Autodesk Inventor part; units mm, degrees
ref_plane "YZ Plane" through (0, 0, 0) normal (1, 0, 0) x (0, 1, 0)
ref_plane "XZ Plane" through (0, 0, 0) normal (0, 1, 0) x (-1, 0, 0)
ref_plane "XY Plane" through (0, 0, 0) normal (0, 0, 1) x (1, 0, 0)
sketch "Sketch1" plane through (0, 0, 0) normal (0, 1, 0) x (-1, 0, 0)
  circle A0 centre (0, 0) radius 335
  dimension "d0" = 670
extrude "Extrusion1" add sketch "Sketch1" along normal blind 10
sketch "Sketch2" plane through (0, 10, 0) normal (0, 1, 0) x (1, 0, 0)
  circle A0 centre (-310, 0) radius 11
  circle A1 centre (0, 0) radius 310 construction
  dimension "d4" = 620
  dimension "d3" = 22
extrude "Cut1" cut sketch "Sketch2" against normal blind 10
pattern_circular "Circular Pattern1" count 20 over 360 about axis through (0, 0, 0) along (0, 1, 0) of "Cut1"
equation "\"d1\" = Thickness"
equation "\"d6\" = Thickness"
equation "\"BendReliefDepth\" = 0.5 * Thickness"
properties part number "PRS 1621 charging hatch D940"
Build history of the part. All positions in model axes, mm. Coordinates: 2 decimals unless noted, no trailing zeros. Write each loop counter-clockwise with the first axis right and the second up, starting at its lowest first coordinate (ties: lowest second). Pieces come first, ordered by that corner, then holes.
1. Band-saw the part on C-C, the plane y = 6.25. Give the number of separate pieces and of enclosed holes in the cut face, and give its area (3 significant figures).
Answer block:
separate pieces: 1
enclosed holes: 20
area: 345,000 mm2
2. Band-saw the part on B-B, the plane x = 0. Give the cut face in (y, z).
Answer block:
outline: (0, -335) - (10, -335) - (10, -321) - (0, -321) - close; (0, -299) - (10, -299) - (10, 299) - (0, 299) - close; (0, 321) - (10, 321) - (10, 335) - (0, 335) - close
3. Drill centre lines: probe 1 along Z at (x, y) = (256, 6.75); probe 2 along X at (y, z) = (4.75, 183.5); probe 3 along X at (y, z) = (8.25, 295.5). Where is each one in solid material? Low to high.
Answer block:
probe 1: z = -216.08 to -191.9, -172.52 to 172.52, 191.9 to 216.08
probe 2: x = -280.27 to -261.72, -239.87 to 239.87, 261.72 to 280.27
probe 3: x = -157.81 to -106.77, -84.82 to 84.82, 106.77 to 157.81
4. Drop flat-ended pins along their axis: pin 1 (6 mm diameter, centred on x = 119, y = 7.5, fed in from +Z); pin 2 (6 mm diameter, centred on x = 90.5, y = 7.5, fed in from -Z); pin 3 (2 mm diameter, centred on x = 109, y = 6, fed in from +Z). Give the stop position or say it passes through.
Answer block:
pin 1: stops at z = 314.28
pin 2: stops at z = -323.37
pin 3: stops at z = 317.11
5. Pull direction Z, two halves, no side cores. Call faces 1 (the flat face through (5, 0, 5)), 2 (the cylindrical face through (265.845, 4.93, 203.842)), 3 (the cylindrical face through (251.463, 5.07, -171.234)), 4 (the cylindrical face through (-181.93, 5.07, 261.79)): released by +Z, released by -Z, zero draft, split by the parting line, or undercut.
Answer block:
face 1: zero draft
face 2: split by the parting line
face 3: undercut
face 4: undercut
6. Band-saw the part on A-A, the plane z = 0. Give the cut face in (x, y).
Answer block:
outline: (-335, 0) - (-321, 0) - (-321, 10) - (-335, 10) - close; (-299, 0) - (299, 0) - (299, 10) - (-299, 10) - close; (321, 0) - (335, 0) - (335, 10) - (321, 10) - close
7. Band-saw the part on D-D, the plane z = -225. Give the cut face in (x, y), and give its area (3 significant figures).
Answer block:
outline: (-248.19, 0) - (248.19, 0) - (248.19, 10) - (-248.19, 10) - close
area: 4,960 mm2
